from build123d import *

# Parameters (mm, degrees)
SKETCH1_W               = 140
SKETCH1_H               = 80
BOSS_EXTRUDE1_DEPTH     = 2
CHAMFER2_SIZE           = 2
SKETCH4_W               = 8
SKETCH4_H               = 10
BOSS_EXTRUDE2_DEPTH     = 7
SKETCH5_R               = 2.05
CUT_EXTRUDE1_DEPTH      = 139.965499445
SKETCH6_W               = 107.8
SKETCH6_H               = 64
CUT_EXTRUDE2_DEPTH      = 5
SKETCH7_R               = 1.65
CUT_EXTRUDE3_DEPTH      = 82.510735624
CUT_EXTRUDE4_DEPTH      = 82.510735624
CUT_EXTRUDE4_DEPTH_BACK = 1
SKETCH8_R               = 3


with BuildPart() as part:
    # Sketch1 → Boss-Extrude1 (new body)
    with BuildSketch(Plane(origin=(0, 0, 0), x_dir=(1, 0, 0), z_dir=(0, 1, 0))):
        Rectangle(SKETCH1_W, SKETCH1_H)
    extrude(amount=BOSS_EXTRUDE1_DEPTH)

    # Sketch3 → Loft1 section 0
    with BuildSketch(Plane(origin=(0, 7, 0), x_dir=(1, 0, 0), z_dir=(0, 1, 0))):
        with BuildLine():
            Line((-63, -33), (63, -33))
            Line((63, -33), (63, 33))
            Line((63, 33), (-63, 33))
            Line((-63, 33), (-63, -33))
        make_face()
    # Sketch2 → Loft1 section 1
    with BuildSketch(Plane(origin=(0, 2, 0), x_dir=(1, 0, 0), z_dir=(0, 1, 0))):
        with BuildLine():
            Line((70, -40), (70, 40))
            Line((70, 40), (-70, 40))
            Line((-70, 40), (-70, -40))
            Line((-70, -40), (70, -40))
        make_face()
    loft()

    # Chamfer2
    chamfer2_edges = [part.edges().sort_by_distance(p)[0] for p in [
        (70, 1, 40),
        (-70, 1, 40),
        (-70, 1, -40),
        (70, 1, -40),
    ]]
    chamfer(chamfer2_edges, length=CHAMFER2_SIZE)

    # Sketch4 → Boss-Extrude2 (add)
    with BuildSketch(Plane.XZ):
        with Locations((-58.9, 20)):
            Rectangle(SKETCH4_W, SKETCH4_H)
        with Locations((-58.9, -20)):
            Rectangle(SKETCH4_W, SKETCH4_H)
        with Locations((58.9, -20)):
            Rectangle(SKETCH4_W, SKETCH4_H)
        with Locations((58.9, 20)):
            Rectangle(SKETCH4_W, SKETCH4_H)
    extrude(amount=BOSS_EXTRUDE2_DEPTH)

    # Sketch5 → Cut-Extrude1 (cut, through all)
    with BuildSketch(Plane.ZY.offset(62.9)):
        with Locations((-20, -3.5)):
            Circle(SKETCH5_R)
        with Locations((20, -3.5)):
            Circle(SKETCH5_R)
    extrude(amount=-CUT_EXTRUDE1_DEPTH, mode=Mode.SUBTRACT)

    # Sketch6 → Cut-Extrude2 (cut)
    with BuildSketch(Plane.XZ):
        Rectangle(SKETCH6_W, SKETCH6_H)
    extrude(amount=-CUT_EXTRUDE2_DEPTH, mode=Mode.SUBTRACT)

    # Sketch7 → Cut-Extrude3 (cut, through all)
    with BuildSketch(Plane.XZ.offset(-5)):
        with Locations(Location((0, 30, 0), (0, 0, 270))):
            Circle(SKETCH7_R)
        with Locations(Location((40, 0, 0), (0, 0, 270))):
            Circle(SKETCH7_R)
        with Locations(Location((25, -20, 0), (0, 0, 270))):
            Circle(SKETCH7_R)
        with Locations(Location((-20, -25, 0), (0, 0, 270))):
            Circle(SKETCH7_R)
        with Locations(Location((-45, 15, 0), (0, 0, 270))):
            Circle(SKETCH7_R)
        with Locations(Location((0, 0, 0), (0, 0, 270))):
            Circle(SKETCH7_R)
    extrude(amount=-CUT_EXTRUDE3_DEPTH, mode=Mode.SUBTRACT)

    # Sketch8 → Cut-Extrude4 (cut, two sides: drawn at the far end of the back side and taken through both)
    with BuildSketch(Plane.XZ.offset(-5).offset(-CUT_EXTRUDE4_DEPTH_BACK)):
        with Locations(Location((0, 30, 0), (0, 0, 41.810314896))):
            Circle(SKETCH8_R)
        with Locations(Location((40, 0, 0), (0, 0, 270))):
            Circle(SKETCH8_R)
        with Locations(Location((25, -20, 0), (0, 0, 270))):
            Circle(SKETCH8_R)
        with Locations(Location((0, 0, 0), (0, 0, 270))):
            Circle(SKETCH8_R)
        with Locations(Location((-45, 15, 0), (0, 0, 270))):
            Circle(SKETCH8_R)
        with Locations(Location((-20, -25, 0), (0, 0, 270))):
            Circle(SKETCH8_R)
    extrude(amount=CUT_EXTRUDE4_DEPTH + CUT_EXTRUDE4_DEPTH_BACK, mode=Mode.SUBTRACT)


solid = part.part
For this review, take the finished solid that the model builds, in its own axes (mm). A direction names the side the tool comes from. Give positions to 0.01 mm unless a question says otherwise; leave off trailing zeros. Use CSV: the item, a comma, the result in double quotes.
Q1. Tool access review of faces 1 (the face through (62.9, -3.5, 17.7)), 2 (the face through (42.53, 5.51, -1.61)), 3 (the face through (-54.9, -3.5, -22.3)), 4 (the face through (-59, -3, -15)): name each direction out of +Z, -Z, +X, -X, +Y, -Y from which nothing blocks a thin tool from reaching the whole face with its end or side.
Conclusion:
face 1,"+Z, -Z, +X, -Y"
face 2,"-Y"
face 3,"+Z, -Z, -Y"
face 4,"+X, -X, -Y"
Q2. Mouldability with a two-part tool opening along X and no side actions: class faces 5 (the face through (-1, 2, -32)), 6 (the face through (-7, 7, -10)), 7 (the face through (62.9, -3.5, -22.3)) as pulls with the +X half, pulls with the -X half, needs draft (parallel to the pull), parting line crosses it, or undercut.
Conclusion:
face 5,"undercut"
face 6,"needs draft"
face 7,"pulls with the +X half"
Q3. For P1, Ø2, axis at y = -3.5, z = -19, coming from the -X side; P2, Ø6, axis at y = -5.5, z = -23, coming from the +X side; P3, Ø4, axis at x = 0, z = 30, coming from the -Y side; P4, Ø10, axis at x = -46.5, z = 5.5, coming from the -Y side, all flat-tipped, find the tip position at first contact; note any pin that passes through.
Conclusion:
P1,"through"
P2,"x = 62.9"
P3,"y = 6"
P4,"y = 5"
Q4. To check wall thickness, follow probe 1 along Z at (x, y) = (-52, 0.5); probe 2 along X at (y, z) = (6.3, 0); probe 3 along Y at (x, z) = (60.75, 20). State the ranges of each line that lie inside material, in increasing order. Write a range as [from, to].
Conclusion:
probe 1,"[-40, -32], [32, 40]"
probe 2,"[-63.98, -1.65], [1.65, 38.35], [41.65, 63.98]"
probe 3,"[-7, -5.55], [-1.45, 7]"
Q5. Take a section at A-A, the plane y = -3.5. State how many separate pieces and enclosed holes the cut face has, then the cut area to 3 significant figures.
Conclusion:
separate pieces,"8"
enclosed holes,"0"
area,"189 mm2"
